Can you work these out from the model? Positions are in its coordinate system, mm. A direction names the side the tool comes from. Round coordinates to 2 decimals unless told otherwise and drop trailing zeros. Loops run counter-clockwise (first coordinate to the right, second up) from the corner with the lowest first, then second, coordinate; pieces in that order, holes last. Notation, with made-up numbers: (-4.75, -21) -> (23.25, -21) arc R27 cw to (23.25, -4) -> close; hole circle Ø5 at (14.5, 72). An arc over 180 degrees is marked (long way). Use a Markdown table: item, result.
Autodesk Inventor part; units mm, degrees
ref_plane "YZ Plane" through (0, 0, 0) normal (1, 0, 0) x (0, 1, 0)
ref_plane "XZ Plane" through (0, 0, 0) normal (0, 1, 0) x (-1, 0, 0)
ref_plane "XY Plane" through (0, 0, 0) normal (0, 0, 1) x (1, 0, 0)
sketch "Эскиз1" plane through (0, 0, 0) normal (0, 0, 1) x (1, 0, 0)
  line L0 (0, 0) -> (17, 0)
  line L1 (17, 0) -> (17, 17)
  line L2 (17, 17) -> (0, 17)
  line L3 (0, 17) -> (0, 0)
  line L4 (-1.5, 18.5) -> (18.5, 18.5)
  line L5 (18.5, 18.5) -> (18.5, -1.5)
  line L6 (18.5, -1.5) -> (-1.5, -1.5)
  line L7 (-1.5, -1.5) -> (-1.5, 18.5)
  dimension "d0" = 20
  dimension "d1" = 1.5
extrude "Выдавливание1" add sketch "Эскиз1" along normal blind 130
sketch "Эскиз2" plane through (-1.5, 18.5, 0) normal (0, 1, 0) x (1, 0, 0)
  line L0 (20, -130) -> (0, -130) construction
  line L1 (20, 0) -> (0, 0) construction
  line L2 (20, 0) -> (20, -130) construction
  circle A0 centre (10, -52.5) radius 2.75
  circle A1 centre (10, -77.5) radius 2.75
  line L3 (10, -77.5) -> (10, -52.5) construction
  point P0 (1.5, 0)
  point P1 (10, -65)
  point P2 (20, -65)
  point P3 (10, 0)
  dimension "d4" = 25
  dimension "d5" = 5.5
extrude "Выдавливание2" cut sketch "Эскиз2" against normal through all
sketch "Эскиз3" plane through (-1.5, -1.5, 0) normal (-1, 0, 0) x (0, 0, 1)
  circle A0 centre (8, 10) radius 2
  circle A1 centre (32, 10) radius 2
  circle A2 centre (98, 10) radius 2
  circle A3 centre (122, 10) radius 2
  point P0 (0, 1.5)
extrude "Выдавливание3" cut sketch "Эскиз3" against normal blind 200
properties part number "side_axis"
1. Which directions (+Z, -Z, +X, -X, +Y, -Y) give clear straight access to the entire face, cutting with the end or side of a thin tool? Please do faces 1 (the flat face through (17.2, 8.6, 130)), 2 (the flat face through (17, 8, 64)).
Answer sheet:
| item | result |
|---|---|
| face 1 | +Z, +X, -X, +Y, -Y |
| face 2 | +Z, -Z |
2. I need wall thicknesses on line 1 (Z direction, x = 8.5, y = 17.65); line 2 (Y direction, x = 9.5, z = 30). Which ranges of each line are inside material? Lowest first, please.
Answer sheet:
| item | result |
|---|---|
| line 1 | z = 0 to 49.75, 55.25 to 74.75, 80.25 to 130 |
| line 2 | y = -1.5 to 0, 17 to 18.5 |
3. I want a section at A-A (z = 98). Please give me the cut outline in (x, y).
Answer sheet:
| item | result |
|---|---|
| outline | (-1.5, -1.5) -> (18.5, -1.5) -> (18.5, 6.5) -> (17, 6.5) -> (17, 0) -> (0, 0) -> (0, 6.5) -> (-1.5, 6.5) -> close; (-1.5, 10.5) -> (0, 10.5) -> (0, 17) -> (17, 17) -> (17, 10.5) -> (18.5, 10.5) -> (18.5, 18.5) -> (-1.5, 18.5) -> close |
4. I want a section at C-C (y = 4). Please give me the cut outline in (x, z).
Answer sheet:
| item | result |
|---|---|
| outline | (-1.5, 0) -> (0, 0) -> (0, 130) -> (-1.5, 130) -> close; (17, 0) -> (18.5, 0) -> (18.5, 130) -> (17, 130) -> close |
5. Will these pins go through, and if not, where does the flat tip stop? pin 1 Ø6.5 at (y, z) = (8.5, 8) entering from +X; pin 2 Ø3 at (y, z) = (8.5, 122) entering from -X.
Answer sheet:
| item | result |
|---|---|
| pin 1 | stops at x = 18.5 |
| pin 2 | passes through |
6. I want a section at D-D (z = 56.5). Please give me the cut outline in (x, y).
Answer sheet:
| item | result |
|---|---|
| outline | (-1.5, -1.5) -> (18.5, -1.5) -> (18.5, 18.5) -> (-1.5, 18.5) -> close; hole (0, 0) -> (17, 0) -> (17, 17) -> (0, 17) -> close |
7. If we mould it in two halves opening along X, with no side actions, what happens to faces 3 (the flat face through (18.5, 9, 64)), 4 (the cylindrical face through (-0.76, 9.101, 99.908)), 5 (the flat face through (-1.5, 8, 64)), 6 (the cylindrical face through (8.142, -0.739, 74.773))? For each: +X half, -X half, draft (parallel to the pull), parting line (faces both ways), or undercut.
Answer sheet:
| item | result |
|---|---|
| face 3 | +X half |
| face 4 | draft |
| face 5 | -X half |
| face 6 | undercut |
8. I want a section at B-B (x = 8.5). Please give me the cut outline in (y, z), plus the area to 3 significant figures.
Answer sheet:
| item | result |
|---|---|
| outline | (-1.5, 0) -> (0, 0) -> (0, 49.75) -> (-1.5, 49.75) -> close; (-1.5, 55.25) -> (0, 55.25) -> (0, 74.75) -> (-1.5, 74.75) -> close; (-1.5, 80.25) -> (0, 80.25) -> (0, 130) -> (-1.5, 130) -> close; (17, 0) -> (18.5, 0) -> (18.5, 49.75) -> (17, 49.75) -> close; (17, 55.25) -> (18.5, 55.25) -> (18.5, 74.75) -> (17, 74.75) -> close; (17, 80.25) -> (18.5, 80.25) -> (18.5, 130) -> (17, 130) -> close |
| area | 357 mm² |
